Geometry: final body of the model. Coordinates: model frame, mm. A direction names the side the tool comes from. Coordinates: 2 decimals unless noted, no trailing zeros. Loops run counter-clockwise (first coordinate to the right, second up) from the corner with the lowest first, then second, coordinate; pieces in that order, holes last. Notation, with made-up numbers: (0.5, 28) -> (50.5, 28) arc R22 cw to (50.5, 35) -> close; hole circle Ø9 at (57.25, 9.25). An arc over 180 degrees is marked (long way). One line per item, written item: value. Start each with the question number.
Item 1: Contact query for flat-ended pins moving along their axis: pin 1 Ø1.7 at (x, z) = (-3.5, -6) entering from +Y; pin 2 Ø4 at (y, z) = (17.5, 2) entering from -X; pin 3 Ø5 at (x, y) = (-1.16, 17) entering from -Z; pin 4 Ø4 at (y, z) = (12.5, -8.5) entering from +X. Output: stop coordinate, or through.
Item 2: Section query A-A on y = 17.75. Return loops of the section in (x, z).
Item 3: Mould query, pull axis Z, two halves, no side actions, for faces 1 (the flat face through (-1, 5, -20.778)), 2 (the flat face through (3.841, 8, -6)), 3 (the cylindrical face through (-4.73, 20.5, 3.63)), 4 (the flat face through (6, 3, -6)). Classes: +Z half, -Z half, draft (parallel to the pull), parting line (faces both ways), or undercut.
Item 4: Ray query, probe 1 along Z at (x, y) = (-3.5, 8.75); probe 2 along X at (y, z) = (17, 3.9); probe 3 along Z at (x, y) = (3.25, 18.5). Return the intervals inside material, ascending. Write a range as from..to.
Item 5: Section query D-D on y = 13. Return loops of the section in (x, z), then the cut area to 3 significant figures.
Item 6: Section query B-B on x = 0. Give the number of separate pieces and of enclosed holes in the cut face, then the cut area to 3 significant figures.
Item 7: Section query C-C on z = -1. Return loops of the section in (x, y), then the cut area to 3 significant figures.
Item 8: Set-up query: faces 5 (the flat face through (-8, 3, -6)), 6 (the flat face through (-1.1, 19.2, -13.635)), 7 (the flat face through (-1, 10, 10)). Return all of +Z, -Z, +X, -X, +Y, -Y with unobstructed straight access to the full face (end or side cutting, diameter ignored); none if empty.
Autodesk Inventor part; units mm, degrees
ref_plane "Work Plane1" through (8.8407, 0, -5.778) normal (0, 0, -1) x (-1, 0, 0)
ref_plane "YZ Plane" through (0, 0, 0) normal (1, 0, 0) x (0, 1, 0)
ref_plane "XZ Plane" through (0, 0, 0) normal (0, 1, 0) x (-1, 0, 0)
sketch "Sketch2" plane through (0, 0, 0) normal (0, 1, 0) x (-1, 0, 0)
  line L0 (11.1593, 9.222) -> (-8.8407, 9.222)
  line L1 (-8.8407, 9.222) -> (-8.8407, -20.778)
  line L2 (-8.8407, -20.778) -> (11.1593, -20.778)
  line L3 (11.1593, -20.778) -> (11.1593, 9.222)
  point P0 (0, 0)
  dimension "d23" = 30
  dimension "d24" = 20
extrude "Extrusion2" add sketch "Sketch2" along normal blind 3
sketch "Sketch3" plane through (0, 3, 0) normal (0, 1, 0) x (1, 0, 0)
  line L0 (8.8407, -9.222) -> (8.8407, 20.778)
  line L1 (8.8407, 20.778) -> (-11.1593, 20.778)
  line L2 (-11.1593, 20.778) -> (-11.1593, -9.222)
  line L3 (-11.1593, -9.222) -> (8.8407, -9.222)
  line L4 (8.8407, -9.222) -> (8.8407, 20.778)
  line L5 (8.8407, 5.778) -> (-11.1593, 5.778)
  line L6 (-11.1593, 20.778) -> (-11.1593, -9.222)
  line L7 (8.8407, -7.222) -> (-11.1593, -7.222)
  line L8 (3.8407, -7.222) -> (-6.1593, -7.222)
  line L9 (-6.1593, -7.222) -> (-6.1593, 5.778)
  line L10 (-6.1593, 5.778) -> (3.8407, 5.778)
  line L11 (3.8407, 5.778) -> (3.8407, -7.222)
  line L12 (8.8407, 20.778) -> (8.8407, -9.222)
  line L13 (-11.1593, -9.222) -> (-11.1593, 20.778)
  line L14 (-11.1593, 20.778) -> (8.8407, 20.778)
  line L15 (8.8407, 20.778) -> (8.8407, -9.222)
  line L16 (-11.1593, -9.222) -> (-11.1593, 20.778)
  line L17 (8.8407, 18.778) -> (-11.1593, 18.778)
  line L18 (3.8407, 18.778) -> (-6.1593, 18.778)
  line L19 (-6.1593, 18.778) -> (-6.1593, 5.778)
  line L20 (3.8407, 5.778) -> (3.8407, 18.778)
  point P0 (0, 0)
  point P1 (8.8407, 18.778)
  point P2 (-11.1593, 18.778)
  point P3 (-6.1593, 18.778)
  point P4 (-6.1593, -7.222)
  dimension "d27" = 2
  dimension "d28" = 10
  dimension "d29" = 5
  dimension "d53" = 20
extrude "Extrusion3" add sketch "Sketch3" along normal blind 3 contours L3 L2 L7 L0 | L7 L9 L5 L11 | L17 L2 L1 L0 | L5 L19 L17 L20
sketch "Sketch4" plane through (0, 6, 0) normal (0, 1, 0) x (1, 0, 0)
  line L0 (8.8407, -7.222) -> (3.8407, -7.222)
  line L1 (8.8407, -9.222) -> (8.8407, -7.222)
  line L2 (8.8407, -7.222) -> (3.8407, -7.222)
  line L3 (3.8407, -7.222) -> (3.8407, 18.778)
  line L4 (3.8407, 18.778) -> (8.8407, 18.778)
  line L5 (8.8407, 18.778) -> (8.8407, 20.778)
  line L6 (8.8407, 20.778) -> (-11.1593, 20.778)
  line L7 (-11.1593, 20.778) -> (-11.1593, 18.778)
  line L8 (-11.1593, 18.778) -> (-6.1593, 18.778)
  line L9 (-6.1593, 18.778) -> (-6.1593, -7.222)
  line L10 (-6.1593, -7.222) -> (-11.1593, -7.222)
  line L11 (-11.1593, -7.222) -> (-11.1593, -9.222)
  line L12 (-11.1593, -9.222) -> (8.8407, -9.222)
  line L13 (8.8407, -7.222) -> (-11.1593, -7.222)
  line L14 (8.8407, -9.222) -> (8.8407, 20.778)
  line L15 (-11.1593, 18.778) -> (-11.1593, -7.222)
  line L16 (-11.1593, 18.778) -> (8.8407, 18.778)
  point P0 (0, 0)
extrude "Extrusion4" add sketch "Sketch4" along normal blind 5 contours L1 L12 L11 L10 L13 L0 | L4 L16 L8 L7 L6 L5
ref_plane "Work Plane1" through (8.8407, 0, -5.778) normal (0, 0, -1) x (-1, 0, 0)
chamfer "Chamfer1" distance 1 angle 80 2 edges at (8.8407, 11, 8.222) (-11.1593, 11, 8.222) measured on face at (2.174, 11, 8.5554)
chamfer "Chamfer2" distance 1 angle 80 2 edges at (8.8407, 11, -19.778) (-11.1593, 11, -19.778) measured on face at (2.174, 11, -19.4446)
sketch "Sketch5" plane through (0, 6, 0) normal (0, 1, 0) x (1, 0, 0)
  line L0 (-6.1593, -7.222) -> (3.8407, -7.222)
  line L1 (3.8407, -7.222) -> (3.8407, 18.778)
  line L2 (3.8407, 18.778) -> (-6.1593, 18.778)
  line L3 (-6.1593, 18.778) -> (-6.1593, -7.222)
  line L4 (3.8407, -5.222) -> (-6.1593, -5.222)
  line L5 (-6.1593, 18.778) -> (-6.1593, -7.222)
  line L6 (-15.1593, 5.778) -> (12.8407, 5.778)
  line L7 (3.8407, 16.778) -> (-6.1593, 16.778)
  point P0 (0, 0)
  point P1 (3.8407, 16.778)
  point P2 (-6.1593, 16.778)
  dimension "d40" = 11
  dimension "d54" = 26
extrude "Extrusion5" add sketch "Sketch5" along normal blind 4 contours L3 L6 L1 L4 | L3 L7 L1 L6
sketch "Sketch6" plane through (0, 10, 0) normal (0, 1, 0) x (1, 0, 0)
  line L0 (-6.1593, -7.222) -> (-6.1593, 18.778)
  line L1 (3.8407, 18.778) -> (3.8407, -7.222)
  line L2 (3.8407, -5.222) -> (3.8407, -2.0792)
  line L3 (3.8407, -2.0792) -> (-6.1593, -2.0792)
  line L4 (-6.1593, -2.0792) -> (-6.1593, -5.222)
  line L5 (3.8407, 16.778) -> (-6.1593, 16.778)
  line L6 (-6.1593, -5.222) -> (3.8407, -5.222)
  line L7 (-6.1593, 5.778) -> (3.8407, 5.778)
  line L8 (3.8407, 13.6351) -> (-6.1593, 13.6351)
  point P0 (0, 0)
  point P1 (-6.1593, -2.0792)
  point P2 (-6.1593, 13.6351)
  point P3 (3.8407, 13.6351)
  dimension "d43" = 22
  dimension "d44" = 3.1429
extrude "Extrusion6" add sketch "Sketch6" along normal blind 12 contours L0 L3 L1 L6 | L0 L5 L1 L8
fillet "Fillet1" radius 5 4 edges at (3.8407, 22, 3.6506) (-6.1593, 22, 3.6506) (-6.1593, 22, -15.2065) (3.8407, 22, -15.2065)
fillet "Fillet2" radius 5 2 edges at (-11.1593, 0, -5.778) (8.8407, 0, -5.778)
fillet "Fillet3" radius 5 2 edges at (-1.1593, 10, -13.6351) (-1.1593, 10, 2.0792)
sketch "Sketch9" plane through (-10.1593, 11, 9.222) normal (0, 0, 1) x (1, 0, 0)
  line L0 (0, 0) -> (18, 0)
  line L1 (4, -5) -> (4, 6)
  line L2 (14, -5) -> (14, 6)
  line L3 (0, 0) -> (18, 0)
  line L4 (4, 0) -> (14, 0)
  line L5 (14, 0) -> (14, -7)
  line L6 (14, -7) -> (4, -7)
  line L7 (4, -7) -> (4, 0)
  line L8 (4, -1) -> (14, -1)
  point P0 (10.1593, -11)
  point P1 (14, -1)
  point P2 (4, -1)
  dimension "d58" = 6
  dimension "d59" = 1
  dimension "d62" = 10
extrude "Extrusion8" add sketch "Sketch9" along normal blind 1 contours L8 L2 L5 L6 L7 L1
sketch "Sketch10" plane through (-6.1593, 6, 5.222) normal (0, 0, 1) x (1, 0, 0)
  circle A0 centre (5, 11) radius 2
  arc A1 (10, 11) -> (0, 11) centre (5, 11) ccw
  point P0 (6.1593, -6)
  dimension "d63" = 4
extrude "Extrusion9" cut sketch "Sketch10" against normal through all
equation "\"d27\" = 0.1 * d53"
equation "\"d28\" = 0.5 * d53"
equation "\"d29\" = 0.25 * d53"
equation "\"d44\" = 0.142857 * d43"
properties part number "uchytka_spojky_medzi_velkym_strednym"
Reply:
1. pin 1: stops at y = 10
1. pin 2: stops at x = -6.16
1. pin 3: stops at z = -16.78
1. pin 4: passes through
2. outline: (-6.1, -16.78) -> (-3.01, -16.78) -> (-3.01, -13.64) -> (-6.1, -13.64) -> close; (-6.1, 2.08) -> (-3.01, 2.08) -> (-3.01, 5.22) -> (-6.1, 5.22) -> close; (0.69, -16.78) -> (3.78, -16.78) -> (3.78, -13.64) -> (0.69, -13.64) -> close; (0.69, 2.08) -> (3.78, 2.08) -> (3.78, 5.22) -> (0.69, 5.22) -> close
3. face 1: -Z half
3. face 2: undercut
3. face 3: draft
3. face 4: undercut
4. probe 1: z = -20.78..-18.78, -16.78..5.22, 7.22..10.22
4. probe 2: x = -6.16..-3.16, 0.84..3.84
4. probe 3: z = -16.78..-13.64, 2.08..5.22
5. outline: (-6.16, -16.78) -> (3.84, -16.78) -> (3.84, -13.22) -> (-6.16, -13.22) -> close; (-6.16, 1.66) -> (3.84, 1.66) -> (3.84, 5.22) -> (-6.16, 5.22) -> close
5. area: 71.2 mm²
6. separate pieces: 3
6. enclosed holes: 0
6. area: 359 mm²
7. outline: (-10.74, 3) arc R5 ccw to (-6.16, 0) -> (3.84, 0) arc R5 ccw to (8.42, 3) -> (3.84, 3) -> (3.84, 10.38) -> (-6.16, 10.38) -> (-6.16, 3) -> close
7. area: 124 mm²
8. face 5: -X, +Y
8. face 6: +X, -X, +Y
8. face 7: +Z, +X, -X, +Y
